Build history of the part. All positions in model axes, mm. Face numbers are marked on the shaded views. A direction names the side the tool comes from. Give positions to 0.01 mm unless a question says otherwise; leave off trailing zeros. Loops run counter-clockwise (first coordinate to the right, second up) from the corner with the lowest first, then second, coordinate; pieces in that order, holes last. Notation, with made-up numbers: (-5, -33.5) -> (31, -33.5) arc R20 ccw to (31, -14.5) -> close; hole circle Ø5 at (52, 18). An arc over 180 degrees is marked (long way). One line per question, with ' | ' between items. Start each with the question number.
(1) Slice it at D-D, the plane y = 2.75. Write the cut outline in (x, z), then the cut area to 3 significant figures.
(2) Slice it at B-B, the plane z = -17. Write the cut outline in (x, y).
(3) 3-axis set-ups, long thin cutter, end or side, ignore diameter. For the marked faces 1, 2 and 3: which of +Z, -Z, +X, -X, +Y, -Y reach the whole face in a straight line?
(4) Drill centre lines: L1, parallel to X at y = 0, z = 13.5; L2, parallel to X at y = -0.75, z = 19; L3, parallel to Z at x = 7.25, y = -10. Where is each one in solid material? Low to high. Write a range as from..to.
(5) Flat gauge pins, fed straight in: pin 1 Ø5 at (x, y) = (5.5, 4) entering from +Z; pin 2 Ø1.9 at (x, y) = (-8.5, 0) entering from -Z; pin 3 Ø2 at (x, z) = (10, 15.5) entering from +Y. Where does each tip first touch, or does it go through?
(6) Slice it at C-C, the plane z = 12.5. Write the cut outline in (x, y).
(7) Slice it at A-A, the plane x = 0. Write the cut outline in (y, z).
```python
from build123d import *

# Parameters (mm, degrees)
SKETCH1_R                           = 13
BOSS_EXTRUDE1_DEPTH                 = 21
SKETCH2_R                           = 5
BOSS_EXTRUDE2_DEPTH                 = 1
SKETCH4_R                           = 5.5
BOSS_EXTRUDE4_DEPTH                 = 1
SKETCH3_R                           = 2
BOSS_EXTRUDE5_DEPTH                 = 9.3
SKETCH5_R                           = 2
BOSS_EXTRUDE6_DEPTH                 = 9.3
F_3_32_0_09375_DIAMETER_HOLE1_D     = 2.38125
F_3_32_0_09375_DIAMETER_HOLE1_DEPTH = 12.7
F_3_32_0_09375_DIAMETER_HOLE1_TIP   = 0.715399675


with BuildPart() as part:
    # Sketch1 → Boss-Extrude1 (new body, symmetric)
    with BuildSketch(Plane(origin=(0, 0, 0), x_dir=(0, 1, 0), z_dir=(0, 0, 1))):
        Circle(SKETCH1_R)
    extrude(amount=BOSS_EXTRUDE1_DEPTH, both=True)

    # Sketch2 → Boss-Extrude2 (add)
    with BuildSketch(Plane.XY.offset(21)):
        Circle(SKETCH2_R)
    extrude(amount=BOSS_EXTRUDE2_DEPTH)

    # Sketch4 → Boss-Extrude4 (add)
    with BuildSketch(Plane(origin=(0, 0, -21), x_dir=(1, 0, 0), z_dir=(0, 0, -1))):
        Circle(SKETCH4_R)
    extrude(amount=BOSS_EXTRUDE4_DEPTH)

    # Sketch3 → Boss-Extrude5 (add)
    with BuildSketch(Plane.XY.offset(22)):
        Circle(SKETCH3_R)
    extrude(amount=BOSS_EXTRUDE5_DEPTH)

    # Sketch5 → Boss-Extrude6 (add)
    with BuildSketch(Plane(origin=(0, 0, -22), x_dir=(1, 0, 0), z_dir=(0, 0, -1))):
        Circle(SKETCH5_R)
    extrude(amount=BOSS_EXTRUDE6_DEPTH)

    # 3/32 (0.09375) Diameter Hole1
    with Locations(Plane.XY.offset(21)):
        with Locations((8.5, 0), (-8.5, 0)):
            Hole(F_3_32_0_09375_DIAMETER_HOLE1_D / 2, depth=F_3_32_0_09375_DIAMETER_HOLE1_DEPTH)
            with Locations((0, 0, -(F_3_32_0_09375_DIAMETER_HOLE1_DEPTH + F_3_32_0_09375_DIAMETER_HOLE1_TIP / 2))):  # 118° drill point
                Cone(0, F_3_32_0_09375_DIAMETER_HOLE1_D / 2, F_3_32_0_09375_DIAMETER_HOLE1_TIP, mode=Mode.SUBTRACT)


solid = part.part
```
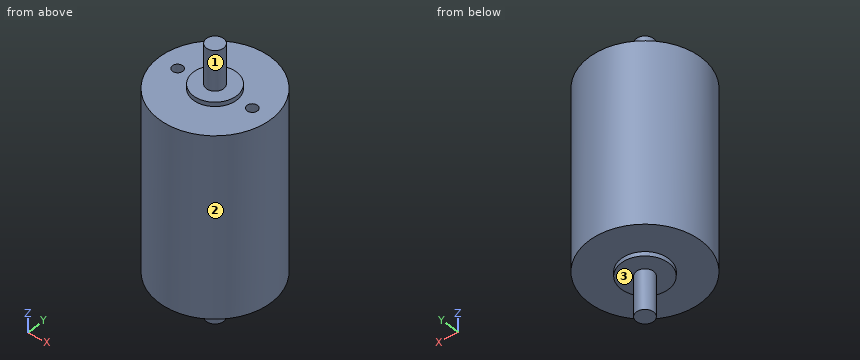
Final values:
1) outline: (-12.71, -21) -> (-4.76, -21) -> (-4.76, -22) -> (4.76, -22) -> (4.76, -21) -> (12.71, -21) -> (12.71, 21) -> (4.18, 21) -> (4.18, 22) -> (-4.18, 22) -> (-4.18, 21) -> (-12.71, 21) -> close | area: 1,090 mm2
2) outline: circle Ø26 at (0, 0)
3) face 1: +Z | face 2: +Z, -Z | face 3: -Z
4) L1: -13..-9.69, -7.31..7.31, 9.69..13 | L2: -12.98..-9.42, -7.58..7.58, 9.42..12.98 | L3: -21..21
5) pin 1: z = 22 | pin 2: z = -21 | pin 3: y = 9.38
6) outline: circle Ø26 at (0, 0); hole circle Ø2.38 at (-8.5, 0); hole circle Ø2.38 at (8.5, 0)
7) outline: (-13, -21) -> (-5.5, -21) -> (-5.5, -22) -> (-2, -22) -> (-2, -31.3) -> (2, -31.3) -> (2, -22) -> (5.5, -22) -> (5.5, -21) -> (13, -21) -> (13, 21) -> (5, 21) -> (5, 22) -> (2, 22) -> (2, 31.3) -> (-2, 31.3) -> (-2, 22) -> (-5, 22) -> (-5, 21) -> (-13, 21) -> close
